from build123d import *

# Parameters (mm, degrees)
BOSS_EXTRUDE1_DEPTH     = 50.8
SKETCH3_W               = 44.45
SKETCH3_H               = 50.8
CUT_EXTRUDE1_DEPTH      = 25.4
SKETCH4_R               = 2.4892
CUT_EXTRUDE2_DEPTH      = 17.78
SKETCH7_W               = 25.4
SKETCH7_H               = 25.4
CUT_EXTRUDE3_DEPTH      = 19.05
CUT_EXTRUDE4_DEPTH      = 159.113724894
CUT_EXTRUDE4_DEPTH_BACK = 159.113724894
SKETCH10_R              = 2.4892
CUT_EXTRUDE5_DEPTH      = 160.257189791
FILLET1_R               = 5.08


with BuildPart() as part:
    # Sketch1 → Boss-Extrude1 (new body)
    with BuildSketch(Plane.XY):
        Polygon((0, 0), (0, -139.7), (-6.35, -139.7), (-6.35, -114.3), (-63.5, -103.787780153), (-43.777988763, -30.184232189), (-6.35, -25.4), (-6.35, 0), align=None)
    extrude(amount=BOSS_EXTRUDE1_DEPTH)

    # Sketch3 → Cut-Extrude1 (cut)
    with BuildSketch(Plane(origin=(-33.299361532, 8.922537031, 0), x_dir=(0, 0, 1), z_dir=(-0.9659258262890682, 0.2588190451025214, 0))):
        with Locations((25.4, -78.586306667)):
            Rectangle(SKETCH3_W, SKETCH3_H)
    extrude(amount=-CUT_EXTRUDE1_DEPTH, mode=Mode.SUBTRACT)

    # Sketch4 → Cut-Extrude2 (cut)
    with BuildSketch(Plane(origin=(-33.299361532, 8.922537031, 0), x_dir=(0, 0, 1), z_dir=(-0.9659258262890682, 0.2588190451025214, 0))):
        with Locations(Location((25.4, -46.836306667, 0), (0, 0, 270))):
            Circle(SKETCH4_R)
        with Locations(Location((25.4, -110.336306667, 0), (0, 0, 270))):
            Circle(SKETCH4_R)
    extrude(amount=-CUT_EXTRUDE2_DEPTH, mode=Mode.SUBTRACT)

    # Sketch7 → Cut-Extrude3 (cut)
    with BuildSketch(Plane(origin=(-8.764845544, 2.348533285, 0), x_dir=(0, 0, 1), z_dir=(-0.9659258262890681, 0.25881904510252124, 0))):
        with Locations((25.4, -78.586306667)):
            Rectangle(SKETCH7_W, SKETCH7_H)
    extrude(amount=-CUT_EXTRUDE3_DEPTH, mode=Mode.SUBTRACT)

    # Sketch9 → Cut-Extrude4 (cut, two sides: drawn at the far end of the back side and taken through both)
    with BuildSketch(Plane(origin=(0, 0, 38.1), x_dir=(-1, 0, 0), z_dir=(0, 0, -1)).offset(-CUT_EXTRUDE4_DEPTH_BACK)):
        Polygon((7.41658953, -66.223254732), (13.990593276, -90.75777072), (26.25785127, -87.470768847), (19.683847524, -62.936252859), align=None)
    extrude(amount=CUT_EXTRUDE4_DEPTH + CUT_EXTRUDE4_DEPTH_BACK, mode=Mode.SUBTRACT)

    # Sketch10 → Cut-Extrude5 (cut, through all)
    with BuildSketch(Plane.ZY.offset(6.35)):
        with Locations(Location((25.4, -12.7, 0), (0, 0, 270))):
            Circle(SKETCH10_R)
        with Locations(Location((12.7, -12.7, 0), (0, 0, 270))):
            Circle(SKETCH10_R)
        with Locations(Location((12.7, -127, 0), (0, 0, 270))):
            Circle(SKETCH10_R)
        with Locations(Location((38.1, -127, 0), (0, 0, 270))):
            Circle(SKETCH10_R)
        with Locations(Location((38.1, -12.7, 0), (0, 0, 270))):
            Circle(SKETCH10_R)
        with Locations(Location((25.4, -127, 0), (0, 0, 270))):
            Circle(SKETCH10_R)
    extrude(amount=-CUT_EXTRUDE5_DEPTH, mode=Mode.SUBTRACT)

    # Fillet1
    # the kernel refuses this fillet: 5.08 mm, written as the material it adds along each edge
    with BuildSketch(Plane(origin=(-6.35, -25.4, 0), x_dir=(0, 1, 0), z_dir=(0, 0, 1))) as fillet1_piece_1:
        with BuildLine():
            CenterArc((FILLET1_R * 0.880311524947, FILLET1_R), FILLET1_R, 187.284330246, 82.715669754)
            Line((-FILLET1_R * 0.111617631295, FILLET1_R * 0.873206668172), (0, 0))
            Line((0, 0), (FILLET1_R * 0.880311524947, 0))
        make_face()
    extrude(amount=50.8)
    with BuildSketch(Plane(origin=(-6.35, -114.3, 0), x_dir=(0, -1, 0), z_dir=(0, 0, 1))) as fillet1_piece_2:
        with BuildLine():
            CenterArc((FILLET1_R * 0.832835540577, -FILLET1_R), FILLET1_R, 90, 79.57746931)
            Line((-FILLET1_R * 0.150664867797, -FILLET1_R * 0.819094094265), (0, 0))
            Line((0, 0), (FILLET1_R * 0.832835540577, 0))
        make_face()
    extrude(amount=50.8)
    # the kernel refuses this fillet: 5.08 mm, written as the material it takes off along each edge
    with BuildSketch(Plane(origin=(-43.777988763, -30.184232189, -8.520486112), x_dir=(0.9919291562424372, 0.12679333182847863, 0), z_dir=(0, 0, 1))) as fillet1_2_piece_1:
        with BuildLine():
            CenterArc((FILLET1_R * 0.670904418298, -FILLET1_R), FILLET1_R, 90, 67.715669754)
            Line((-FILLET1_R * 0.254409042496, -FILLET1_R * 0.620796889158), (0, 0))
            Line((0, 0), (FILLET1_R * 0.670904418298, 0))
        make_face()
    extrude(amount=67.840972225, mode=Mode.SUBTRACT)
    with BuildSketch(Plane(origin=(-63.5, -103.787780153, -13.757429812), x_dir=(0.983500408373109, -0.18090590573535092, 0), z_dir=(0, 0, 1))) as fillet1_2_piece_2:
        with BuildLine():
            CenterArc((FILLET1_R * 1.0832621899, FILLET1_R), FILLET1_R, 175.42253069, 94.57746931)
            Line((FILLET1_R * 0.0864518515073, FILLET1_R * 1.07980695008), (0, 0))
            Line((0, 0), (FILLET1_R * 1.0832621899, 0))
        make_face()
    extrude(amount=78.314859623, mode=Mode.SUBTRACT)


solid = part.part
Geometry check sheet. Reference: the model listing, model coordinates, mm. A direction names the side the tool comes from. Coordinates: 2 decimals unless noted, no trailing zeros. Order: outer loops, then holes, each group sorted by start corner. A loop starts at its lowest first (then second) coordinate and runs counter-clockwise, first axis right, second up. Notation, with made-up numbers: (29, 62) -> (70, 62) arc R13 ccw to (70, 81) -> close; hole circle Ø4 at (64.25, 73). An arc over 180 degrees is marked (long way). Use a Markdown table: item, result. Add a question column.
1. Cross-section at A-A (x = -4). Enter the section's corners in (y, z), and give its area (3 significant figures).
2. Set-up check for faces 5 (the face through (-3.22, -12.38, 27.87)), 6 (the face through (-44.673, -102.222, 25.435)), 7 (the face through (-6.35, -132, 25)), 8 (the face through (-6.35, -8, 25)): record each of +Z, -Z, +X, -X, +Y, -Y from which the full face is reachable in a straight line by a thin tool's end or side.
3. Mould release check, pull along Y, two halves, no side actions. Record for faces 1 (the face through (0, -69, 25)), 2 (the face through (-23.02, -75.38, 6.44)), 3 (the face through (-33.97, -109.22, 25.04)), 4 (the face through (-34.969, -45.692, 25.089)): pulls with the +Y half, pulls with the -Y half, needs draft (parallel to the pull), parting line crosses it, or undercut.
4. Cross-section at D-D (y = -76.5). Enter the section's corners in (x, z) (3 decimals).
5. Go/stop test with flat-tipped pins: pin 1 Ø23.5 at (y, z) = (-133.5, 24) entering from -X; pin 2 Ø3 at (x, z) = (-30, 33) entering from -Y; pin 3 Ø12 at (x, z) = (-42, 14.5) entering from -Y; pin 4 Ø12 at (y, z) = (-38.5, 15) entering from +X. Record where each tip stops, or that it passes through.
6. Cross-section at B-B (y = -127). Enter the section's corners in (x, z).
7. Material ranges on L1, parallel to Y at x = -4, z = 38; L2, parallel to Z at x = -2, y = -12; L3, parallel to X at y = -21.5, z = 46, recorded low to high.
Filled sheet:
| question | item | result |
|---|---|---|
| 1 | outline | (-139.7, 0) -> (0, 0) -> (0, 50.8) -> (-139.7, 50.8) -> close; hole circle Ø4.98 at (-127, 12.7); hole circle Ø4.98 at (-127, 25.4); hole circle Ø4.98 at (-127, 38.1); hole circle Ø4.98 at (-12.7, 12.7); hole circle Ø4.98 at (-12.7, 25.4); hole circle Ø4.98 at (-12.7, 38.1) |
| 1 | area | 6,980 mm2 |
| 2 | face 5 | +X, -X |
| 2 | face 6 | none |
| 2 | face 7 | +Z, -Z, -X, -Y |
| 2 | face 8 | +Z, -Z, -X, +Y |
| 3 | face 1 | needs draft |
| 3 | face 2 | undercut |
| 3 | face 3 | pulls with the -Y half |
| 3 | face 4 | undercut |
| 4 | outline | (-56.188, 0) -> (-23.318, 0) -> (-23.318, 12.7) -> (-29.892, 12.7) -> (-29.892, 3.175) -> (-56.188, 3.175) -> close; (-56.188, 47.625) -> (-29.892, 47.625) -> (-29.892, 38.1) -> (-23.318, 38.1) -> (-23.318, 50.8) -> (-56.188, 50.8) -> close; (-10.17, 0) -> (0, 0) -> (0, 50.8) -> (-10.17, 50.8) -> close |
| 5 | pin 1 | x = -6.35 |
| 5 | pin 2 | y = -110.23 |
| 5 | pin 3 | y = -108.85 |
| 5 | pin 4 | x = 0 |
| 6 | outline | (-6.35, 0) -> (0, 0) -> (0, 10.21) -> (-6.35, 10.21) -> close; (-6.35, 15.19) -> (0, 15.19) -> (0, 22.91) -> (-6.35, 22.91) -> close; (-6.35, 27.89) -> (0, 27.89) -> (0, 35.61) -> (-6.35, 35.61) -> close; (-6.35, 40.59) -> (0, 40.59) -> (0, 50.8) -> (-6.35, 50.8) -> close |
| 7 | L1 | -139.7 to -129.49, -124.51 to -15.19, -10.21 to 0 |
| 7 | L2 | 0 to 10.31, 15.09 to 23.01, 27.79 to 35.71, 40.49 to 50.8 |
| 7 | L3 | -6.38 to 0 |
